Autodesk Inventor part; units mm, degrees
ref_plane "YZ Plane" through (0, 0, 0) normal (1, 0, 0) x (0, 1, 0)
ref_plane "XZ Plane" through (0, 0, 0) normal (0, 1, 0) x (-1, 0, 0)
ref_plane "XY Plane" through (0, 0, 0) normal (0, 0, 1) x (1, 0, 0)
sketch "Szkic32" plane through (0, 0, 0) normal (0, 0, 1) x (1, 0, 0)
  line L0 (0, 0) -> (10, 0)
  line L1 (10, 0) -> (15.9865, -2.9108)
  line L2 (10, 0) -> (16.6566, 0) construction
  line L3 (10, 0) -> (20.0005, -4.8625)
  line L4 (20.0005, -4.8625) -> (20.0005, -7.9995)
  line L5 (20.0005, -7.9995) -> (18.0005, -7.9995)
  line L6 (0, 0) -> (0, -2)
  line L7 (0, -2) -> (10, -2)
  line L8 (10, -2) -> (18.0005, -5.89)
  line L9 (10, -2) -> (18.8961, -2) construction
  line L10 (18.0005, -5.89) -> (18.0005, -7.9995)
  dimension "d102" = 10
  dimension "d103" = 25.93
  dimension "d104" = 11.12
  dimension "d105" = 3.137
  dimension "d106" = 2
  dimension "d107" = 2
  dimension "d108" = 10
  dimension "d109" = 25.93
extrude "Wyciągnięcie proste35" add sketch "Szkic32" along normal blind 24.3
sketch "Szkic33" plane through (0, 0, 24.3) normal (0, 0, 1) x (1, 0, 0)
  line L0 (10, 0) -> (0, 0)
  line L1 (0, 0) -> (0, -2)
  line L2 (0, -2) -> (10, -2)
  line L3 (0, 0) -> (10, 0)
  line L4 (10, 0) -> (10, -2)
  line L5 (10, -2) -> (0, -2)
  line L6 (0, -2) -> (0, 0)
  line L7 (10, -2) -> (15.396, -4.6236)
  line L8 (10, -2) -> (18.0005, -5.89)
  line L9 (15.396, -4.6236) -> (15.396, -2.6236)
  line L10 (20.0005, -4.8625) -> (10, 0)
  line L11 (10, 0) -> (15.396, -2.6236)
  dimension "d112" = 6
extrude "Wyciągnięcie proste36" add sketch "Szkic33" along normal blind 20.2
sketch "Szkic34" plane through (0, 0, 44.5) normal (0, 0, 1) x (1, 0, 0)
  line L0 (10, 0) -> (0, 0)
  line L1 (0, -2) -> (10, -2)
  line L2 (0, 0) -> (10, 0)
  line L3 (10, 0) -> (10, -2)
  line L4 (10, -2) -> (0, -2)
  line L5 (0, -2) -> (0, 0)
extrude "Wyciągnięcie proste37" add sketch "Szkic34" along normal blind 17.5
sketch "Szkic36" plane through (0, 0, 62) normal (0, 0, 1) x (1, 0, 0)
  line L0 (15.396, -2.6236) -> (10, 0)
  line L1 (15.396, -4.6236) -> (15.396, -2.6236)
  line L2 (10, -2) -> (15.396, -4.6236)
  line L3 (0, -2) -> (10, -2)
  line L4 (10, 0) -> (0, 0)
  line L5 (0, 0) -> (0, -2)
  line L6 (10, 0) -> (15.396, -2.6236)
  line L7 (15.396, -2.6236) -> (15.396, -4.6236)
extrude "Wyciągnięcie proste38" add sketch "Szkic36" along normal blind 20
sketch "Szkic37" plane through (0, 0, 82) normal (0, 0, 1) x (1, 0, 0)
  line L0 (10, 0) -> (0, 0)
  line L1 (0, -2) -> (10, -2)
  line L2 (0, 0) -> (10, 0)
  line L3 (10, 0) -> (10, -2)
  line L4 (10, -2) -> (0, -2)
  line L5 (0, -2) -> (0, 0)
extrude "Wyciągnięcie proste39" add sketch "Szkic37" along normal blind 17.5
sketch "Szkic38" plane through (0, 0, 99.5) normal (0, 0, 1) x (1, 0, 0)
  line L0 (15.396, -2.6236) -> (10, 0)
  line L1 (15.396, -4.6236) -> (15.396, -2.6236)
  line L2 (10, -2) -> (15.396, -4.6236)
  line L3 (0, -2) -> (10, -2)
  line L4 (10, 0) -> (0, 0)
  line L5 (10, 0) -> (0, 0)
  line L6 (0, 0) -> (0, -2)
  line L7 (0, -2) -> (10, -2)
  line L8 (10, -2) -> (10, 0)
extrude "Wyciągnięcie proste40" add sketch "Szkic38" along normal blind 20.2
sketch "Szkic39" plane through (0, 0, 119.7) normal (0, 0, 1) x (1, 0, 0)
  line L0 (15.396, -2.6236) -> (15.396, -4.6236)
  line L1 (15.396, -4.6236) -> (18.0005, -5.89)
  line L2 (18.0005, -5.89) -> (18.0005, -7.9995)
  line L3 (18.0005, -7.9995) -> (20.0005, -7.9995)
  line L4 (20.0005, -7.9995) -> (20.0005, -4.8625)
  line L5 (20.0005, -4.8625) -> (15.396, -2.6236)
  line L6 (0, 0) -> (0, -2)
  line L7 (0, -2) -> (10, -2)
  line L8 (10, -2) -> (15.396, -4.6236)
  line L9 (15.396, -4.6236) -> (15.396, -2.6236)
  line L10 (15.396, -2.6236) -> (10, 0)
  line L11 (10, 0) -> (0, 0)
extrude "Wyciągnięcie proste41" add sketch "Szkic39" along normal blind 24.3
sketch "Szkic40" plane through (0, 0, 0) normal (0, 1, 0) x (1, 0, 0)
  line L0 (0, 0) -> (0, -144)
  line L1 (0, -17.3) -> (6.3, -17.3)
  line L2 (6.3, -17.3) -> (6.3, -23.6)
  line L3 (6.3, -23.6) -> (0, -23.6)
  line L4 (0, -23.6) -> (0, -17.3)
  line L5 (10, 0) -> (0, 0)
  line L6 (0, -126.7) -> (6.3, -126.7)
  line L7 (6.3, -126.7) -> (6.3, -120.4)
  line L8 (6.3, -120.4) -> (0, -120.4)
  line L9 (0, -120.4) -> (0, -126.7)
  line L10 (10, -144) -> (0, -144)
  point P0 (0, -120.4)
  point P1 (0, -23.6)
  dimension "d125" = 6.3
  dimension "d126" = 6.3
  dimension "d127" = 17.3
  dimension "d128" = 6.3
  dimension "d129" = 6.3
  dimension "d130" = 17.3
extrude "Wyciągnięcie proste42" cut sketch "Szkic40" against normal blind 2
properties part number "prrzod"
Work out the finished part from the listing and answer in its coordinate system (mm). A direction names the side the tool comes from. Round coordinates to 2 decimals unless told otherwise and drop trailing zeros. Loops run counter-clockwise (first coordinate to the right, second up) from the corner with the lowest first, then second, coordinate; pieces in that order, holes last. Notation, with made-up numbers: (56.5, 77) -> (88.5, 77) arc R20 cw to (88.5, 99) -> close; hole circle Ø5 at (64, 68.25). An arc over 180 degrees is marked (long way). Use one line per item in the form item = value.
(1) Find section B-B on z = 15. Give the vertices of the cut face in (x, y).
Answer list:
outline = (0, -2) -> (10, -2) -> (18, -5.89) -> (18, -8) -> (20, -8) -> (20, -4.86) -> (15.99, -2.91) -> (10, 0) -> (0, 0) -> close
(2) Straight lines are drawn through the part: line 1 (Z direction, x = 15.5, y = -3.25); line 2 (Z direction, x = 4.75, y = -1.5); line 3 (Y direction, x = 5.5, z = 89.5). For each, find the intervals that lie inside material, in ascending order.
Answer list:
line_1 = 0 to 24.3, 119.7 to 144
line_2 = 0 to 17.3, 23.6 to 120.4, 126.7 to 144
line_3 = -2 to 0
(3) Find section A-A on x = 1.25. Give the vertices of the cut face in (y, z), then the cut area to 3 significant figures.
Answer list:
outline = (-2, 0) -> (0, 0) -> (0, 17.3) -> (-2, 17.3) -> close; (-2, 23.6) -> (0, 23.6) -> (0, 120.4) -> (-2, 120.4) -> close; (-2, 126.7) -> (0, 126.7) -> (0, 144) -> (-2, 144) -> close
area = 263 mm2
(4) Find section D-D on z = 105. Give the vertices of the cut face in (x, y), then the cut area to 3 significant figures.
Answer list:
outline = (0, -2) -> (10, -2) -> (15.4, -4.62) -> (15.4, -2.62) -> (10, 0) -> (0, 0) -> close
area = 30.8 mm2
(5) For a pull along Z with two mould halves and no side action, classify faces 1 (the flat face through (13, -2, 44.5)), 2 (the flat face through (5, 0, 71)), 3 (the flat face through (11, -2, 0)), 4 (the flat face through (11, -2, 144)) as released by +Z, released by -Z, zero draft, split by the parting line, or undercut.
Answer list:
face_1 = undercut
face_2 = zero draft
face_3 = released by -Z
face_4 = released by +Z
(6) Find section C-C on x = 12. Give the vertices of the cut face in (y, z), then the cut area to 3 significant figures.
Answer list:
outline = (-2.97, 0) -> (-0.97, 0) -> (-0.97, 44.5) -> (-2.97, 44.5) -> close; (-2.97, 62) -> (-0.97, 62) -> (-0.97, 82) -> (-2.97, 82) -> close; (-2.97, 99.5) -> (-0.97, 99.5) -> (-0.97, 144) -> (-2.97, 144) -> close
area = 218 mm2
(7) Flat-ended cylindrical pins translate along their axes: P1, Ø10, axis at x = 8, z = 105.5, coming from the -Y side; P2, Ø4, axis at x = 12.5, z = 63, coming from the +Y side; P3, Ø0.6, axis at y = -4, z = 32, coming from the +X side. Find the tip coordinate at first contact, or state that the pin passes through.
Answer list:
P1 = -3.46
P2 = -0.24
P3 = 15.4
(8) A tool of negligible diameter and unlimited length cuts with its end or side. For faces 5 (the flat face through (20, -6, 12)), 6 (the flat face through (5, -2, 71)), 7 (the flat face through (18, -5, 119.7)), from which of +Z, -Z, +X, -X, +Y, -Y can it reach the whole face along a straight path? Write none if from no direction.
Answer list:
face_5 = +Z, -Z, +X, +Y, -Y
face_6 = +Z, -Z, -X, -Y
face_7 = +X, +Y, -Y
